```python
from build123d import *

# Parameters (mm, degrees)
CYLINDER129_R             = 1.75
CYLINDER129_DEPTH         = 26
CYLINDER131_R             = 1.75
CYLINDER131_DEPTH         = 26
BOX066_W                  = 7
BOX066_H                  = 48
BOX066_DEPTH              = 1
CYLINDER132_R             = 1.5
CYLINDER132_DEPTH         = 10
CYLINDER130_R             = 5
CYLINDER130_DEPTH         = 1
CYLINDER128_R             = 17.5
CYLINDER128_DEPTH         = 22
FUSION092_ROLL_ANGLE      = 90.000432
FUSION092_PITCH_ANGLE     = 62.999717
FUSION092_PLACEMENT_ANGLE = 90.000641


with BuildPart() as cylinder129:
    # Cylinder129 → Cylinder129 (new body)
    with BuildSketch(Plane(origin=(0, 21, 0), x_dir=(1, 0, 0), z_dir=(0, 0, 1))):
        Circle(CYLINDER129_R)
    extrude(amount=CYLINDER129_DEPTH)


with BuildPart() as cylinder131:
    # Cylinder131 → Cylinder131 (new body)
    with BuildSketch(Plane(origin=(0, -21, 0), x_dir=(1, 0, 0), z_dir=(0, 0, 1))):
        Circle(CYLINDER131_R)
    extrude(amount=CYLINDER131_DEPTH)


with BuildPart() as cut183:
    # Box066 → Box066 (new body)
    with BuildSketch(Plane(origin=(-3.4, -23.6, 22), x_dir=(1, 0, 0), z_dir=(0, 0, 1))):
        with Locations((3.5, 24)):
            Rectangle(BOX066_W, BOX066_H)
    extrude(amount=BOX066_DEPTH)

    # Cut182: cut Cylinder131
    add(cylinder131.part, mode=Mode.SUBTRACT)

    # Cut183: cut Cylinder129
    add(cylinder129.part, mode=Mode.SUBTRACT)


with BuildPart() as cut183_1:
    # Cut183 placement: moved
    add(cut183.part.moved(Location((0, 0, -1))))


with BuildPart() as cylinder132:
    # Cylinder132 → Cylinder132 (new body)
    with BuildSketch(Plane.XY.offset(23)):
        Circle(CYLINDER132_R)
    extrude(amount=CYLINDER132_DEPTH)


with BuildPart() as cylinder130:
    # Cylinder130 → Cylinder130 (new body)
    with BuildSketch(Plane.XY.offset(22)):
        Circle(CYLINDER130_R)
    extrude(amount=CYLINDER130_DEPTH)


with BuildPart() as fusion092:
    # Cylinder128 → Cylinder128 (new body)
    with BuildSketch(Plane.XY):
        Circle(CYLINDER128_R)
    extrude(amount=CYLINDER128_DEPTH)

    # Fusion092: union Cut183, Cylinder132, Cylinder130
    add(cut183_1.part)
    add(cylinder132.part)
    add(cylinder130.part)


with BuildPart() as fusion092_1:
    # Fusion092 roll: moved
    add(fusion092.part.rotate(Axis((0, 0, 0), (1, 0, 0)), FUSION092_ROLL_ANGLE))


with BuildPart() as fusion092_2:
    # Fusion092 pitch: moved
    add(fusion092_1.part.rotate(Axis((0, 0, 0), (0, 1, 0)), FUSION092_PITCH_ANGLE))


with BuildPart() as fusion092_3:
    # Fusion092 placement: moved
    add(fusion092_2.part.moved(Location((77.100367, 12.900556, 96.792998))).rotate(Axis((77.100367, 12.900556, 96.792998), (0, 0, 1)), FUSION092_PLACEMENT_ANGLE))


solid = fusion092_3.part
```
Check sheet for the modelled part. Datum: model origin and axes. Units: mm. Round coordinates to 2 decimals unless told otherwise and drop trailing zeros. Write item = value, one per line.
Q1. Thickness scan on line 1 along Y through (x, z) = (94.5, 97); line 2 along X through (y, z) = (1.5, 107); line 3 along X through (y, z) = (11, 97). Record the ranges inside material, lowest first.
Computed:
line_1 = -4.6 to 30.4
line_2 = 77.1 to 99.1
line_3 = 77.1 to 100.1
Q2. Draft check along Z on faces 1 (the face through (105.03, 12.03, 95.57)), 2 (the face through (98.593, -5.674, 85.514)). Enter one of: pulls with the +Z half, pulls with the -Z half, needs draft (parallel to the pull), parting line crosses it, or undercut.
Computed:
face_1 = parting line crosses it
face_2 = undercut
Q3. Go/stop test with flat-tipped pins: pin 1 (2 mm diameter, centred on x = 91, z = 104.5, fed in from +Y); pin 2 (10.5 mm diameter, centred on y = 21, z = 105.5, fed in from +X); pin 3 (3 mm diameter, centred on x = 95, y = 3.5, fed in from +Z). Record where each tip stops, or that it passes through.
Computed:
pin_1 = 29.06
pin_2 = 99.1
pin_3 = 112.41
